from build123d import *

# Parameters (mm, degrees)
F0_R     = 1.5
F1_DEPTH = 4
F0_R_2   = 11
F0_R_3   = 4
F2_DEPTH = 2
F3_R     = 5
F3_R_2   = 4
F4_DEPTH = 2
F5_SIZE  = 0.2


with BuildPart() as f1:
    # F0 (on Top) → F1 (new body)
    with BuildSketch(Plane.XY):
        with Locations((-8, 0)):
            Circle(F0_R)
    extrude(amount=F1_DEPTH)



with BuildPart() as f1b:
    # F0 (on Top) → F1, piece 2 (new body)
    with BuildSketch(Plane.XY):
        with Locations((-4, 6.9282032303)):
            Circle(F0_R)
    extrude(amount=F1_DEPTH)


with BuildPart() as f1c:
    # F0 (on Top) → F1, piece 3 (new body)
    with BuildSketch(Plane.XY):
        with Locations((4, 6.9282032303)):
            Circle(F0_R)
    extrude(amount=F1_DEPTH)


with BuildPart() as f1d:
    # F0 (on Top) → F1, piece 4 (new body)
    with BuildSketch(Plane.XY):
        with Locations((8, 0)):
            Circle(F0_R)
    extrude(amount=F1_DEPTH)


with BuildPart() as f1e:
    # F0 (on Top) → F1, piece 5 (new body)
    with BuildSketch(Plane.XY):
        with Locations((4, -6.9282032303)):
            Circle(F0_R)
    extrude(amount=F1_DEPTH)


with BuildPart() as f1f:
    # F0 (on Top) → F1, piece 6 (new body)
    with BuildSketch(Plane.XY):
        with Locations((-4, -6.9282032303)):
            Circle(F0_R)
    extrude(amount=F1_DEPTH)


with BuildPart() as f1_1:
    add(f1.part)

    add(f1b.part)  # F2 merges F1b

    add(f1c.part)  # F2 merges F1c

    add(f1d.part)  # F2 merges F1d

    add(f1e.part)  # F2 merges F1e

    add(f1f.part)  # F2 merges F1f
    # F0 (on Top) → F2 (join)
    with BuildSketch(Plane.XY):
        Circle(F0_R_2)
        with Locations((-4, -6.9282032303)):
            Circle(F0_R, mode=Mode.SUBTRACT)
        with Locations((4, -6.9282032303)):
            Circle(F0_R, mode=Mode.SUBTRACT)
        with Locations((-8, 0)):
            Circle(F0_R, mode=Mode.SUBTRACT)
        with Locations((-4, 6.9282032303)):
            Circle(F0_R, mode=Mode.SUBTRACT)
        Circle(F0_R_3, mode=Mode.SUBTRACT)
        with Locations((8, 0)):
            Circle(F0_R, mode=Mode.SUBTRACT)
        with Locations((4, 6.9282032303)):
            Circle(F0_R, mode=Mode.SUBTRACT)
        with Locations((4, -6.9282032303)):
            Circle(F0_R)
        with Locations((8, 0)):
            Circle(F0_R)
        with Locations((4, 6.9282032303)):
            Circle(F0_R)
        with Locations((-4, 6.9282032303)):
            Circle(F0_R)
        with Locations((-8, 0)):
            Circle(F0_R)
        with Locations((-4, -6.9282032303)):
            Circle(F0_R)
    extrude(amount=-F2_DEPTH)

    # F3 (on face) → F4 (join)
    with BuildSketch(Plane(origin=(0, 0, -2), x_dir=(1, 0, 0), z_dir=(0, 0, -1))):
        Circle(F3_R)
        Circle(F3_R_2, mode=Mode.SUBTRACT)
    extrude(amount=F4_DEPTH)

    # F5
    f5_edges = [f1_1.edges().sort_by_distance(p)[0] for p in [
        (-11, 0, 0),
        (-5.5, -6.928203, 0),
        (-9.5, 0, 0),
        (2.5, -6.928203, 0),
        (-4, 0, 0),
        (6.5, 0, 0),
        (-5.5, 6.928203, 0),
        (2.5, 6.928203, 0),
        (6.5, 0, 4),
        (2.5, -6.928203, 4),
        (-5.5, -6.928203, 4),
        (-9.5, 0, 4),
        (-5.5, 6.928203, 4),
        (2.5, 6.928203, 4),
        (-4, 0, -4),
        (-5, 0, -4),
        (-5, 0, -2),
        (-11, 0, -2),
    ]]
    chamfer(f5_edges, length=F5_SIZE)


solid = f1_1.part
Model file for the job. Use its own axes, mm. A direction names the side the tool comes from. Give positions to 0.01 mm unless a question says otherwise; leave off trailing zeros. Order: outer loops, then holes, each group sorted by start corner. A loop starts at its lowest first (then second) coordinate and runs counter-clockwise, first axis right, second up. Notation, with made-up numbers: (-38, 62) - (-24, 62) arc R14 cw to (-24, 66) - close; hole circle Ø6 at (42, 28.5). An arc over 180 degrees is marked (long way). Write item = value, one per line. Start each with the question number.
1. Two-plate mould, pull along Y, no slides. Class faces 1 (the flat face through (5, 3, -2)), 2 (the cylindrical face through (-4.2, -5.44, 1.97)): pulls with the +Y half, pulls with the -Y half, needs draft (parallel to the pull), parting line crosses it, or undercut.
2. Cut at C-C, the plane z = -3.5. List the corners of the cut face in (x, y), and give its area (3 significant figures).
3. Drop flat-ended pins along their axis: P1, Ø4, axis at x = -4, z = -1, coming from the -Y side; P2, Ø4, axis at y = 8, z = 3, coming from the +X side; P3, Ø5, axis at x = -1.5, y = 7.5, coming from the -Z side. Give the stop position or say it passes through.
4. Cut at A-A, the plane x = 0. List the corners of the cut face in (y, z), and give its area (3 significant figures).
5. Cut at B-B, the plane z = 2.75. List the corners of the cut face in (x, y).
6. Which spindle directions (+Z, -Z, +X, -X, +Y, -Y) get a long thin tool onto all of the face, cutting with end or side? Do faces 3 (the flat face through (-4, -7, 4)), 4 (the cylindrical face through (-2.57, 7.38, 1.97)). Say none if no direction does.
7. Probe line 1 along Y through (x, z) = (0, -2.85); line 2 along Y through (x, z) = (0, -0.7). List the from-to ranges inside material, lowest first.
Taken from the geometry:
q1.face_1 = needs draft
q1.face_2 = undercut
q2.outline = circle Ø10 at (0, 0); hole circle Ø8 at (0, 0)
q2.area = 28.3 mm²
q3.P1 = -10.82
q3.P2 = 5.5
q3.P3 = -2.05
q4.outline = (-11, -1.8) - (-10.8, -2) - (-5.2, -2) - (-5, -2.2) - (-5, -3.8) - (-4.8, -4) - (-4.2, -4) - (-4, -3.8) - (-4, -0.2) - (-4.2, 0) - (-10.8, 0) - (-11, -0.2) - close; (4, -3.8) - (4.2, -4) - (4.8, -4) - (5, -3.8) - (5, -2.2) - (5.2, -2) - (10.8, -2) - (11, -1.8) - (11, -0.2) - (10.8, 0) - (4.2, 0) - (4, -0.2) - close
q4.area = 31.8 mm²
q5.outline = circle Ø3 at (-8, 0); circle Ø3 at (-4, -6.93); circle Ø3 at (-4, 6.93); circle Ø3 at (4, -6.93); circle Ø3 at (4, 6.93); circle Ø3 at (8, 0)
q6.face_3 = +Z, +X, -X, +Y, -Y
q6.face_4 = +Z
q7.line_1 = -5 to -4, 4 to 5
q7.line_2 = -11 to -4, 4 to 11
